Can you work these out from the drawing? Everything is in mm from the part's minimum corner. Round coordinates to 2 decimals unless told otherwise and drop trailing zeros. Loops run counter-clockwise (first coordinate to the right, second up) from the corner with the lowest first, then second, coordinate; pieces in that order, holes last. Notation, with made-up numbers: (22.25, 23) - (79.25, 23) arc R12 cw to (79.25, 34) - close; hole circle Ø10 at (-1.5, -7.75). An arc over 180 degrees is marked (long way). Return JSON: item names as keys, results as strings. Group by question number.
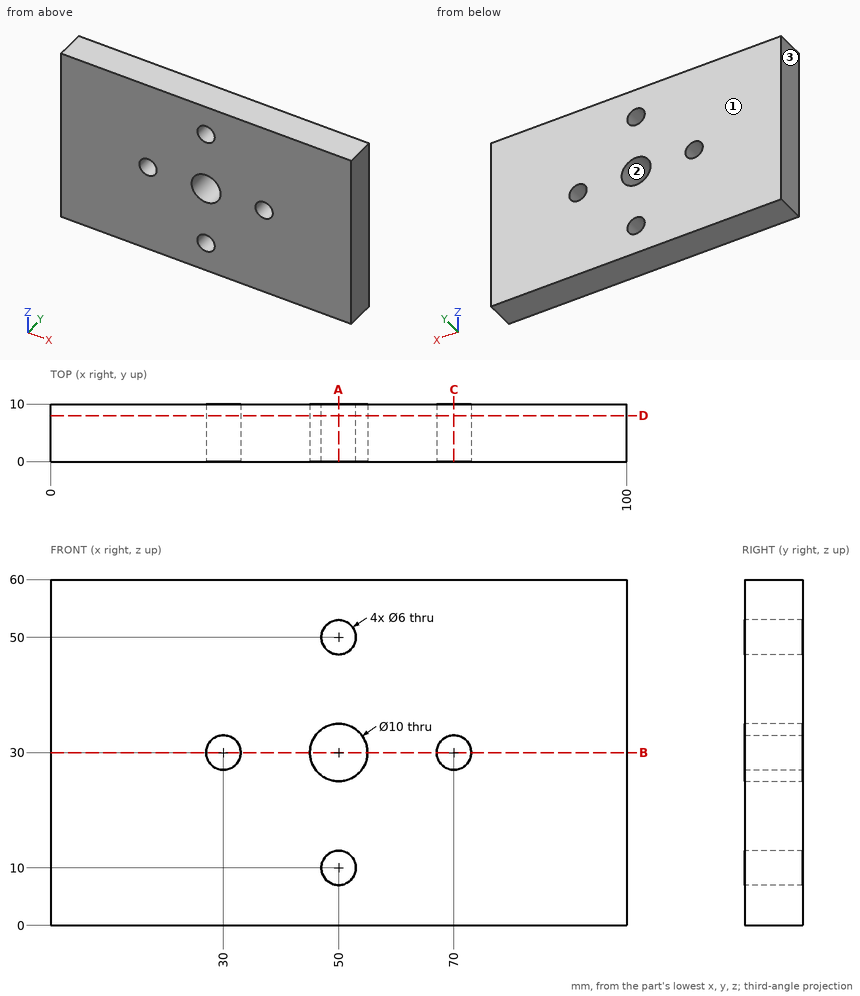
Q1. If we mould it in two halves opening along X, with no side actions, what happens to the marked faces 1, 2 and 3? For each: +X half, -X half, draft (parallel to the pull), parting line (faces both ways), or undercut.
Q2. Imagine slicing it at C-C, the plane x = 70. List the corners of the cut face in (y, z) for me.
Q3. Imagine slicing it at D-D, the plane y = 8. List the corners of the cut face in (x, z) for me, and give its area (3 significant figures).
Q4. Will this pin go through, and if not, where does the flat tip stop? pin 1 Ø5.5 at (x, z) = (50, 10) entering from -Y.
Q5. Imagine slicing it at A-A, the plane x = 50. List the corners of the cut face in (y, z) for me, and give its area (3 significant figures).
Q6. Please list where these lines run through material, in increasing order: line 1 (Z direction, x = 50, y = 7); line 2 (X direction, y = 4, z = 30); line 3 (X direction, y = 3.5, z = 50).
Q7. Imagine slicing it at B-B, the plane z = 30. List the corners of the cut face in (x, y) for me.
Output values:
{
 "1": {"face 1": "draft", "face 2": "undercut", "face 3": "-X half"},
 "2": {"outline": "(0, 0) - (10, 0) - (10, 27) - (0, 27) - close; (0, 33) - (10, 33) - (10, 60) - (0, 60) - close"},
 "3": {"outline": "(0, 0) - (100, 0) - (100, 60) - (0, 60) - close; hole circle Ø6 at (30, 30); hole circle Ø10 at (50, 30); hole circle Ø6 at (50, 10); hole circle Ø6 at (50, 50); hole circle Ø6 at (70, 30)", "area": "5,810 mm^2"},
 "4": {"pin 1": "passes through"},
 "5": {"outline": "(0, 0) - (10, 0) - (10, 7) - (0, 7) - close; (0, 13) - (10, 13) - (10, 25) - (0, 25) - close; (0, 35) - (10, 35) - (10, 47) - (0, 47) - close; (0, 53) - (10, 53) - (10, 60) - (0, 60) - close", "area": "380 mm^2"},
 "6": {"line 1": "z = 0 to 7, 13 to 25, 35 to 47, 53 to 60", "line 2": "x = 0 to 27, 33 to 45, 55 to 67, 73 to 100", "line 3": "x = 0 to 47, 53 to 100"},
 "7": {"outline": "(0, 0) - (27, 0) - (27, 10) - (0, 10) - close; (33, 0) - (45, 0) - (45, 10) - (33, 10) - close; (55, 0) - (67, 0) - (67, 10) - (55, 10) - close; (73, 0) - (100, 0) - (100, 10) - (73, 10) - close"}
}
